For this review, use the dimensioned drawing (mm, ordinates from the lowest corner) and the shaded views. A direction names the side the tool comes from. Coordinates: 2 decimals unless noted, no trailing zeros. Write each loop counter-clockwise with the first axis right and the second up, starting at its lowest first coordinate (ties: lowest second). Pieces come first, ordered by that corner, then holes. Notation, with made-up numbers: (87, 11.5) - (127, 11.5) arc R5 ccw to (127, 19.5) - close; hole circle Ø10 at (-9.75, 89). An arc over 180 degrees is marked (long way). Answer as a JSON object with one key per item and string values.
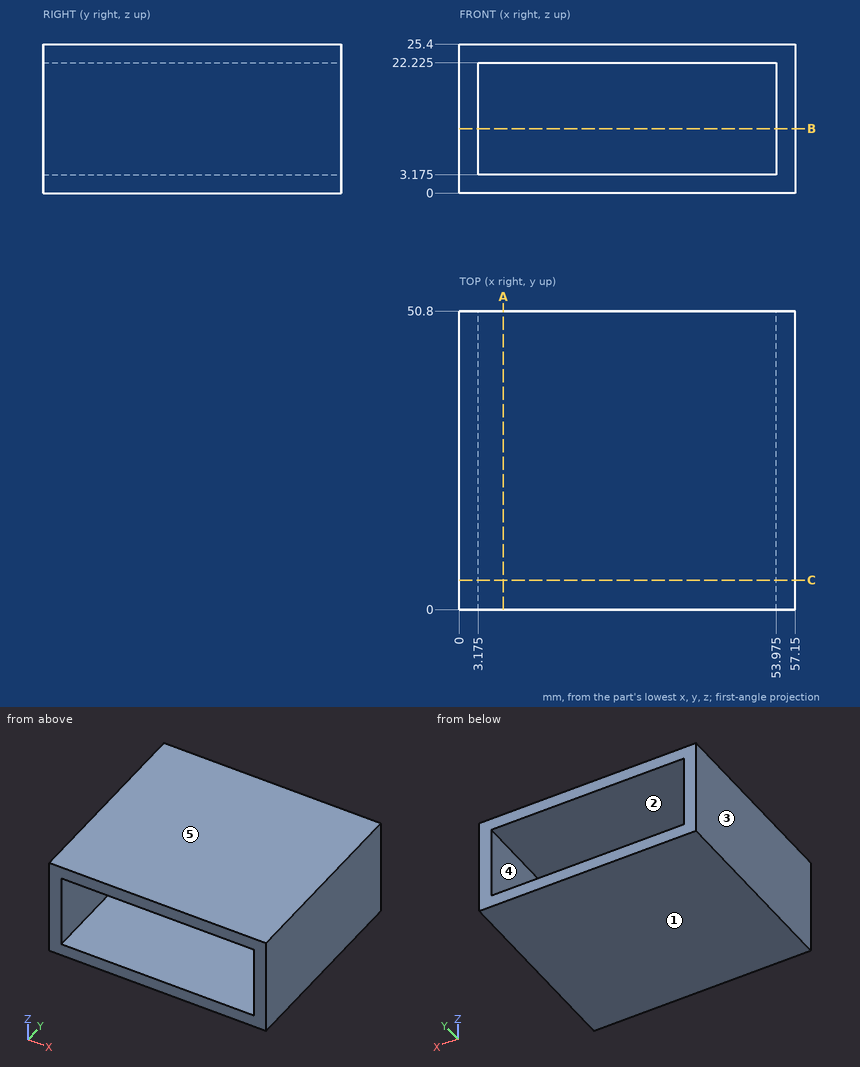
(1) Tool access review of the marked faces 4 and 5: name each direction out of +Z, -Z, +X, -X, +Y, -Y from which nothing blocks a thin tool from reaching the whole face with its end or side.
Solved:
{"face 4": "+Y, -Y", "face 5": "+Z, +X, -X, +Y, -Y"}
(2) Take a section at B-B, the plane z = 11. Write out the cut boundary in (x, y) (3 decimals).
Solved:
{"outline": "(0, 0) - (3.175, 0) - (3.175, 50.8) - (0, 50.8) - close; (53.975, 0) - (57.15, 0) - (57.15, 50.8) - (53.975, 50.8) - close"}
(3) To check wall thickness, follow line 1 (X direction, y = 21.5, z = 9.75) (3 decimals); line 2 (Z direction, x = 49, y = 37) (3 decimals). State the ranges of each line that lie inside material, in increasing order. Write a range as from..to.
Solved:
{"line 1": "x = 0..3.175, 53.975..57.15", "line 2": "z = 0..3.175, 22.225..25.4"}
(4) Take a section at C-C, the plane y = 5. Write out the cut boundary in (x, z) (3 decimals).
Solved:
{"outline": "(0, 0) - (57.15, 0) - (57.15, 25.4) - (0, 25.4) - close; hole (3.175, 3.175) - (53.975, 3.175) - (53.975, 22.225) - (3.175, 22.225) - close"}
(5) Take a section at A-A, the plane x = 7.5. Write out the cut boundary in (y, z) (3 decimals).
Solved:
{"outline": "(0, 0) - (50.8, 0) - (50.8, 3.175) - (0, 3.175) - close; (0, 22.225) - (50.8, 22.225) - (50.8, 25.4) - (0, 25.4) - close"}
(6) The part is to be moulded in two halves that separate along Z. For the marked faces 1, 2 and 3, say which applies: pulls with the +Z half, pulls with the -Z half, needs draft (parallel to the pull), parting line crosses it, or undercut.
Solved:
{"face 1": "pulls with the -Z half", "face 2": "undercut", "face 3": "needs draft"}
